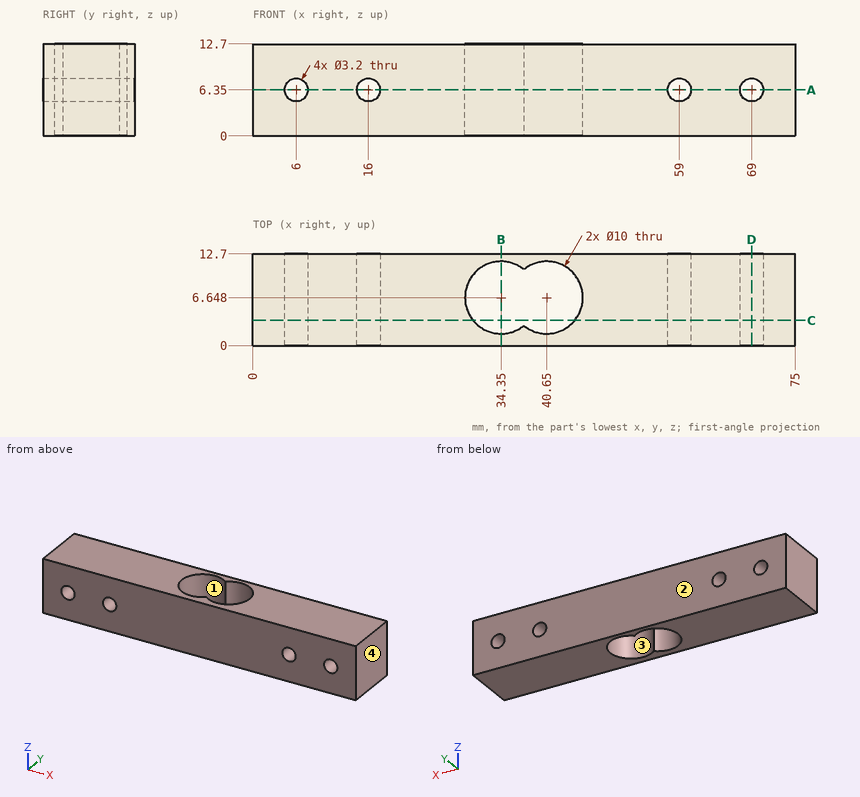
Here's the drawing with two shaded views (mm, measured from the low corner). I have some questions. Give positions to 0.01 mm unless a question says otherwise; leave off trailing zeros. Order: outer loops, then holes, each group sorted by start corner. A loop starts at its lowest first (then second) coordinate and runs counter-clockwise, first axis right, second up. Notation, with made-up numbers: M 68.25,25.5 L 106.25,25.5 A29 ccw 106.25,53.5 Z; hole C -11,30.25 d8. An arc over 180 degrees is marked long. One line per item, written item: value.
1) I want a section at B-B, the plane x = 34.35. List the corners of the cut face in (y, z) for me, plus the area to 3 significant figures.
Answer sheet:
outline: M 0,0 L 1.65,0 L 1.65,12.7 L 0,12.7 Z; M 11.65,0 L 12.7,0 L 12.7,12.7 L 11.65,12.7 Z
area: 34.3 mm^2
2) For P1, Ø2, axis at x = 43.5, y = 6.5, coming from the +Z side, with a flat end and sliding along its axis, tell me the tip position at first contact or that it passes through.
Answer sheet:
P1: passes through
3) We'd pull the mould along X, two halves only. Please class the marked faces 1, 2, 3 and 4: released by +X, released by -X, zero draft, split by the parting line, or undercut.
Answer sheet:
face 1: undercut
face 2: zero draft
face 3: undercut
face 4: released by +X
4) I want a section at C-C, the plane y = 3.5. List the corners of the cut face in (x, z) for me, plus the area to 3 significant figures.
Answer sheet:
outline: M 0,0 L 30.47,0 L 30.47,12.7 L 0,12.7 Z; M 44.53,0 L 75,0 L 75,12.7 L 44.53,12.7 Z; hole C 6,6.35 d3.2; hole C 16,6.35 d3.2; hole C 59,6.35 d3.2; hole C 69,6.35 d3.2
area: 742 mm^2
5) I want a section at D-D, the plane x = 69. List the corners of the cut face in (y, z) for me.
Answer sheet:
outline: M 0,0 L 12.7,0 L 12.7,4.75 L 0,4.75 Z; M 0,7.95 L 12.7,7.95 L 12.7,12.7 L 0,12.7 Z
6) Please list where these lines run through material, in increasing order: line 1 along X through (y, z) = (8, 6.35); line 2 along X through (y, z) = (3.5, 6.35) (1 decimal); line 3 along Y through (x, z) = (40.5, 9.75).
Answer sheet:
line 1: x = 0 to 4.4, 7.6 to 14.4, 17.6 to 29.54, 45.46 to 57.4, 60.6 to 67.4, 70.6 to 75
line 2: x = 0 to 4.4, 7.6 to 14.4, 17.6 to 30.5, 44.5 to 57.4, 60.6 to 67.4, 70.6 to 75
line 3: y = 0 to 1.65, 11.65 to 12.7
7) I want a section at A-A, the plane z = 6.35. Count the separate pieces of the cut face and the enclosed holes in it, plus the area to 3 significant figures.
Answer sheet:
separate pieces: 5
enclosed holes: 1
area: 653 mm^2
